```python
from build123d import *

# Parameters (mm, degrees)
F0_W        = 80
F0_H        = 80
F0_R        = 5
F1_DEPTH    = 12
F2_R        = 20
F3_W        = 80
F3_H        = 10
F4_DEPTH    = 95
F6_DEPTH    = 25
F7_T1_DEPTH = 10
F8_R        = 20
F8_R_2      = 12.5
F9_DEPTH    = 35
F11_DEPTH   = 5


# Not quite as in the source:
# - a fillet or chamfer that OpenCascade refuses, or shapes differently, is made with other operations: its cross-section is extruded or revolved along the edge and cut away or added


with BuildPart() as f1:
    # F0 (on Front) → F1 (new body)
    with BuildSketch(Plane.XZ):
        Rectangle(F0_W, F0_H)
        with Locations((-25, 20)):
            Circle(F0_R, mode=Mode.SUBTRACT)
        with Locations((25, 20)):
            Circle(F0_R, mode=Mode.SUBTRACT)
    extrude(amount=F1_DEPTH)

    # F2
    f2_edges = [f1.edges().sort_by_distance(p)[0] for p in [
        (40, -6, 40),
        (-40, -6, 40),
    ]]
    fillet(f2_edges, radius=F2_R)

    # F3 (on face) → F4 (join)
    with BuildSketch(Plane.XZ.offset(12)):
        with Locations((0, -35)):
            Rectangle(F3_W, F3_H)
    extrude(amount=F4_DEPTH)

    # F5 (on face) → F6 (cut)
    with BuildSketch(Plane.XY.offset(-30)):
        with BuildLine():
            Line((-40, -107), (0, -107))
            ThreePointArc((0, -107), (-21.9575829196, -97.4417355508), (-29.9234068918, -74.857636822))
            Line((-29.9234068918, -74.857636822), (-29.9234068918, -12))
            Line((-29.9234068918, -12), (-40, -12))
            Line((-40, -12), (-40, -107))
        make_face()
        with BuildLine():
            ThreePointArc((29.9234068918, -74.857636822), (29.9808456081, -75.9281340463), (30, -77))
            ThreePointArc((30, -77), (21.2132034356, -98.2132034356), (0, -107))
            Line((0, -107), (40, -107))
            Line((40, -107), (40, -12))
            Line((40, -12), (29.9234068918, -12))
            Line((29.9234068918, -12), (29.9234068918, -74.857636822))
        make_face()
    extrude(amount=-F6_DEPTH, mode=Mode.SUBTRACT)

    # F7: fillet of radius 15 on 2 edges, made by hand

    # F7_s2 → F7_t1 (join)
    with BuildSketch(Plane.XY.offset(-40)):
        with BuildLine():
            ThreePointArc((-40, -12), (-32.6994324281, -17.4756259202), (-29.9234068918, -26.1689824821))
            Line((-29.9234068918, -26.1689824821), (-29.9234068918, -12))
            Line((-29.9234068918, -12), (-40, -12))
        make_face()
        with BuildLine():
            ThreePointArc((40, -12), (32.6994324281, -17.4756259202), (29.9234068918, -26.1689824821))
            Line((29.9234068918, -26.1689824821), (29.9234068918, -12))
            Line((29.9234068918, -12), (40, -12))
        make_face()
    extrude(amount=F7_T1_DEPTH)

    # F8 (on face) → F9 (join)
    with BuildSketch(Plane.XY.offset(-30)):
        with Locations((0, -77)):
            Circle(F8_R)
        with Locations((0, -77)):
            Circle(F8_R_2, mode=Mode.SUBTRACT)
    extrude(amount=F9_DEPTH)

    # F10 (on Right) → F11 (join, symmetric)
    with BuildSketch(Plane.YZ):
        with BuildLine():
            Line((-57.3581678378, -29.785791263), (-12.3581678378, -29.785791263))
            Line((-12.3581678378, -29.785791263), (-12.3581678378, 40.214208737))
            ThreePointArc((-12.3581678378, 40.214208737), (-29.3813213863, 15.6725490137), (-57.3581678378, 5.214208737))
            Line((-57.3581678378, 5.214208737), (-57.3581678378, -29.785791263))
        make_face()
    extrude(amount=F11_DEPTH, both=True)


solid = f1.part
```
Geometry check sheet. Reference: the model listing, model coordinates, mm. A direction names the side the tool comes from. Give positions to 0.01 mm unless a question says otherwise; leave off trailing zeros. Write each loop counter-clockwise with the first axis right and the second up, starting at its lowest first coordinate (ties: lowest second). Pieces come first, ordered by that corner, then holes. Notation, with made-up numbers: (-12.75, 55.25) -> (28.25, 55.25) arc R24 ccw to (28.25, 66.25) -> close; hole circle Ø8 at (36, -26). An arc over 180 degrees is marked (long way). One line per question, with ' | ' between items.
Item 1: Access from +Z, -Z, +X, -X, +Y, -Y to the whole of each face (thin tool, end or side, straight path). Record for faces 1 (the cylindrical face through (33.986, -6.084, 34.297)), 2 (the flat face through (-5, -35, -10)), 3 (the flat face through (0, -77, -30)), 4 (the flat face through (5, -35, -10)).
Determined:
face 1: +Z, +X, +Y, -Y | face 2: +Z, -X | face 3: +Z | face 4: +Z, +X
Item 2: Sectioned sample at D-D, the plane x = 0. Record the boundary of the cut face in (y, z).
Determined:
outline: (-107, -40) -> (0, -40) -> (0, 40) -> (-12, 40) -> (-12, -30) -> (-57, -30) -> (-57, -29.79) -> (-12.36, -29.79) -> (-12.36, 40.21) arc R50 cw to (-57.36, 5.21) -> (-57.36, 5) -> (-64.5, 5) -> (-64.5, -30) -> (-89.5, -30) -> (-89.5, 5) -> (-97, 5) -> (-97, -30) -> (-107, -30) -> close
Item 3: Scan lines: line 1 along Y through (x, z) = (0, -16); line 2 along Z through (x, y) = (4.5, -24.5); line 3 along Z through (x, y) = (28.5, -20). Record each from-to range of solid material in increasing order.
Determined:
line 1: -97 to -89.5, -64.5 to -12.36, -12 to 0 | line 2: -40 to -30, -29.79 to 20.01 | line 3: -40 to -30
Item 4: Draft check along X on faces 5 (the cylindrical face through (32.775, -17.37, -35.07)), 6 (the cylindrical face through (-29, -6, 17)), 7 (the flat face through (0, -12.358, 5)). Enter one of: released by +X, released by -X, zero draft, split by the parting line, or undercut.
Determined:
face 5: released by +X | face 6: undercut | face 7: zero draft
Item 5: Depth check by flat-ended pin: pin 1 (11.5 mm diameter, centred on x = -25, z = 20, fed in from -Y); pin 2 (5 mm diameter, centred on y = -78, z = -3, fed in from -X); pin 3 (6 mm diameter, centred on x = 25, z = 20, fed in from -Y); pin 4 (3 mm diameter, centred on x = 1.5, z = -29.5, fed in from -Y). Enter the tip coordinate at first touch or a pass-through.
Determined:
pin 1: y = -12 | pin 2: x = -20 | pin 3: through | pin 4: y = -107
Item 6: Sectioned sample at C-C, the plane x = -25. Record the boundary of the cut face in (y, z).
Determined:
outline: (-93.58, -40) -> (0, -40) -> (0, 15) -> (-12, 15) -> (-12, -30) -> (-93.58, -30) -> close; (-12, 25) -> (0, 25) -> (0, 39.36) -> (-12, 39.36) -> close
Item 7: Sectioned sample at B-B, the plane y = -34. Record the boundary of the cut face in (x, z).
Determined:
outline: (-29.92, -40) -> (29.92, -40) -> (29.92, -30) -> (-29.92, -30) -> close; (-5, -29.79) -> (5, -29.79) -> (5, 12.48) -> (-5, 12.48) -> close
Item 8: Sectioned sample at A-A, the plane z = -20.5. Record the boundary of the cut face in (x, y).
Determined:
outline: (-40, -12) -> (40, -12) -> (40, 0) -> (-40, 0) -> close; (-5, -57.36) -> (-3.77, -57.36) arc R20 ccw (long way) to (3.77, -57.36) -> (5, -57.36) -> (5, -12.36) -> (-5, -12.36) -> close; hole circle Ø25 at (0, -77)
